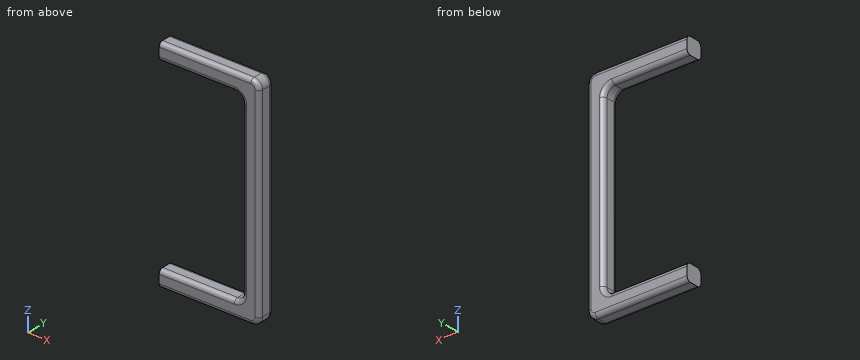
from build123d import *

# Parameters (mm, degrees)
F3_DEPTH = 3.175
F4_R     = 1.5875


# Not quite as in the source:
# - the program builds the solid bodies; features that only make, move or delete a surface that nothing else refers to are left out


with BuildPart() as f3:
    # F2 (on Front) → F3 (new body, symmetric)
    with BuildSketch(Plane.XZ):
        with BuildLine():
            Line((72.3697372794, 95.25), (37.3974703252, 95.25))
            Line((37.3974703252, 95.25), (37.3974703252, 88.9))
            Line((37.3974703252, 88.9), (66.0197372794, 88.9))
            ThreePointArc((66.0197372794, 88.9), (68.2648013097, 87.9700640303), (69.1947372794, 85.725))
            Line((69.1947372794, 85.725), (69.1947372794, 22.225))
            ThreePointArc((69.1947372794, 22.225), (68.2648013097, 19.9799359697), (66.0197372794, 19.05))
            Line((66.0197372794, 19.05), (37.3974703252, 19.05))
            Line((37.3974703252, 19.05), (37.3974703252, 12.7))
            Line((37.3974703252, 12.7), (72.3697372794, 12.7))
            ThreePointArc((72.3697372794, 12.7), (74.6148013097, 13.6299359697), (75.5447372794, 15.875))
            Line((75.5447372794, 15.875), (75.5447372794, 92.075))
            ThreePointArc((75.5447372794, 92.075), (74.6148013097, 94.3200640303), (72.3697372794, 95.25))
        make_face()
    extrude(amount=F3_DEPTH, both=True)

    # F4
    f4_edges = [f3.edges().sort_by_distance(p)[0] for p in [
        (54.883604, -3.175, 12.7),
        (54.883604, 3.175, 12.7),
        (51.708604, 3.175, 19.05),
        (51.708604, -3.175, 19.05),
    ]]
    fillet(f4_edges, radius=F4_R)


solid = f3.part
Could you check a few things on this model? Use its own coordinates, in mm. Coordinates: 2 decimals unless noted, no trailing zeros. Write each loop counter-clockwise with the first axis right and the second up, starting at its lowest first coordinate (ties: lowest second). Pieces come first, ordered by that corner, then holes. Notation, with made-up numbers: (26, 19) - (78, 19) arc R9 cw to (78, 30) - close; hole circle Ø7 at (50, 9.25). An arc over 180 degrees is marked (long way). Put each result on its own line as item: value. Start each with the question number.
Q1. I want a section at B-B on y = 0. Write out the boundary of the cut face in (x, z) (3 decimals), plus the area to 3 significant figures.
Q2. I'm going to push flat-ended pins straight in: P1, Ø1.6, axis at y = 0, z = 56.5, coming from the -X side; P2, Ø2, axis at x = 49.5, y = 2.5, coming from the -Z side. Where does each tip first touch, or does it pass through?
Q3. Please list where these lines run through material, in increasing order: L1, parallel to Z at x = 59, y = 1; L2, parallel to X at y = 1, z = 52.
Q4. I want a section at C-C on z = 49. Write out the boundary of the cut face in (x, y) (1 decimal), plus the area to 3 significant figures.
Checks:
1. outline: (37.397, 12.7) - (72.37, 12.7) arc R3.175 ccw to (75.545, 15.875) - (75.545, 92.075) arc R3.175 ccw to (72.37, 95.25) - (37.397, 95.25) - (37.397, 88.9) - (66.02, 88.9) arc R3.175 cw to (69.195, 85.725) - (69.195, 22.225) arc R3.175 cw to (66.02, 19.05) - (37.397, 19.05) - close
1. area: 928 mm²
2. P1: x = 69.19
2. P2: z = 12.7
3. L1: 12.7 to 19.05, 88.9 to 95.25
3. L2: 69.19 to 75.54
4. outline: (69.2, -1.6) arc R1.6 ccw to (70.8, -3.2) - (74, -3.2) arc R1.6 ccw to (75.5, -1.6) - (75.5, 1.6) arc R1.6 ccw to (74, 3.2) - (70.8, 3.2) arc R1.6 ccw to (69.2, 1.6) - close
4. area: 38.2 mm²
